```python
from build123d import *

# Parameters (mm, degrees)
SALIENTE_EXTRUIR1_DEPTH = 10
REDONDEO1_R             = 2
CROQUIS4_R              = 1.75
SALIENTE_EXTRUIR2_DEPTH = 2
REDONDEO3_R             = 1
REDONDEO4_R             = 0.9


with BuildPart() as part:
    # Croquis2 → Saliente-Extruir1 (new body)
    with BuildSketch(Plane.XY):
        with BuildLine():
            Line((-10.4, 0), (10.4, 0))
            Line((10.4, 0), (10.4, 38))
            Line((10.4, 38), (6.4, 38))
            Line((6.4, 38), (6.4, 36))
            ThreePointArc((6.4, 36), (7.814213562, 35.414213562), (8.4, 34))
            Line((8.4, 34), (8.4, 1.5))
            Line((8.4, 1.5), (-8.4, 1.5))
            Line((-8.4, 1.5), (-8.4, 34))
            ThreePointArc((-8.4, 34), (-7.814213562, 35.414213562), (-6.4, 36))
            Line((-6.4, 36), (-6.4, 38))
            Line((-6.4, 38), (-10.4, 38))
            Line((-10.4, 38), (-10.4, 0))
        make_face()
    extrude(amount=SALIENTE_EXTRUIR1_DEPTH)

    # Redondeo1
    redondeo1_edges = [part.edges().sort_by_distance(p)[0] for p in [
        (-8.4, 1.5, 5),
        (8.4, 1.5, 5),
    ]]
    fillet(redondeo1_edges, radius=REDONDEO1_R)

    # Croquis4 → Saliente-Extruir2 (add)
    # profile 1 of 2: a face of its own
    with BuildSketch(Plane.XZ):
        with BuildLine():
            Line((-10.4, 10), (-15.4, 10))
            ThreePointArc((-15.4, 10), (-20.4, 5), (-15.4, 0))
            Line((-15.4, 0), (-10.4, 0))
            Line((-10.4, 0), (-10.4, 10))
        make_face()
        with Locations((-15.4, 5)):
            Circle(CROQUIS4_R, mode=Mode.SUBTRACT)
    # profile 2 of 2: a face of its own
    with BuildSketch(Plane.XZ):
        with BuildLine():
            Line((10.4, 0), (15.4, 0))
            ThreePointArc((15.4, 0), (20.4, 5), (15.4, 10))
            Line((15.4, 10), (10.4, 10))
            Line((10.4, 10), (10.4, 0))
        make_face()
        with Locations(Location((15.4, 5, 0), (0, 0, 180))):
            Circle(CROQUIS4_R, mode=Mode.SUBTRACT)
    extrude(amount=-SALIENTE_EXTRUIR2_DEPTH)

    # Redondeo3
    redondeo3_edges = [part.edges().sort_by_distance(p)[0] for p in [
        (-10.4, 2, 5),
        (10.4, 2, 5),
    ]]
    fillet(redondeo3_edges, radius=REDONDEO3_R)

    # Redondeo4
    redondeo4_edges = [part.edges().sort_by_distance(p)[0] for p in [
        (-10.4, 20.5, 0),
        (-7.814213562, 35.414213562, 0),
        (8.4, 18.75, 0),
        (7.814213562, 35.414213562, 0),
        (7.814213562, 35.414213562, 10),
        (8.4, 18.75, 10),
        (-7.814213562, 35.414213562, 10),
        (0, 1.5, 0),
        (0, 1.5, 10),
        (-8.4, 18.75, 0),
        (-8.4, 18.75, 10),
        (-8.4, 38, 10),
        (7.814213562, 2.085786438, 0),
        (7.814213562, 2.085786438, 10),
        (-7.814213562, 2.085786438, 0),
        (-7.814213562, 2.085786438, 10),
        (-10.4, 20.5, 10),
        (-13.4, 2, 0),
        (-20.4, 2, 5),
        (13.4, 2, 10),
        (20.4, 2, 5),
        (10.4, 20.5, 10),
        (10.4, 20.5, 0),
        (13.4, 2, 0),
        (-13.4, 2, 10),
        (10.692893219, 2.292893219, 0),
        (10.692893219, 2.292893219, 10),
        (-10.692893219, 2.292893219, 10),
        (-10.692893219, 2.292893219, 0),
        (8.4, 38, 10),
    ]]
    fillet(redondeo4_edges, radius=REDONDEO4_R)


solid = part.part
```
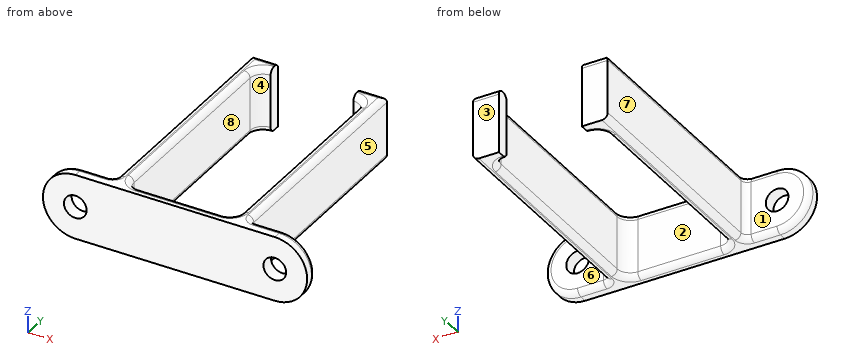
Here's how the part is built. I have some questions about the finished solid (model axes, mm). Face numbers are marked on the shaded views. A direction names the side the tool comes from. Give positions to 0.01 mm unless a question says otherwise; leave off trailing zeros. Loops run counter-clockwise (first coordinate to the right, second up) from the corner with the lowest first, then second, coordinate; pieces in that order, holes last. Notation, with made-up numbers: M -2.5,-10 L 48.5,-10 A23 ccw 48.5,26 Z; hole C -8.5,-1.75 d3. An arc over 180 degrees is marked long. Return JSON: item names as keys, results as strings.
Item 1: Imagine slicing it at A-A on y = 6.5. List the corners of the cut face in (x, z) for me.
A:
{"outline": "M -10.4,0.9 A0.9 ccw -9.5,0 L -9.3,0 A0.9 ccw -8.4,0.9 L -8.4,9.1 A0.9 ccw -9.3,10 L -9.5,10 A0.9 ccw -10.4,9.1 Z; M 8.4,0.9 A0.9 ccw 9.3,0 L 9.5,0 A0.9 ccw 10.4,0.9 L 10.4,9.1 A0.9 ccw 9.5,10 L 9.3,10 A0.9 ccw 8.4,9.1 Z"}
Item 2: Thinking about a two-plate mould opening in Y: for the marked faces 6, 7 and 8, which applies, released by +Y, released by -Y, zero draft, split by the parting line, or undercut?
A:
{"face 6": "released by +Y", "face 7": "zero draft", "face 8": "undercut"}
Item 3: On a 3-axis mill with a long thin cutter (end or side, diameter ignored), from which of +Z, -Z, +X, -X, +Y, -Y can I reach the whole of each face in a straight line? I mean the marked faces 1, 2, 3, 4 and 5. Say none if no direction works.
A:
{"face 1": "+Z, -Z, -X, +Y", "face 2": "+Z, -Z, +Y", "face 3": "+Z, -Z, +X, -X, +Y", "face 4": "+Z, -Z", "face 5": "+Z, -Z, +X, +Y"}
Item 4: Imagine slicing it at D-D on x = 4.5. List the corners of the cut face in (y, z) for me.
A:
{"outline": "M 0,0 L 0.6,0 A0.9 ccw 1.5,0.9 L 1.5,9.1 A0.9 ccw 0.6,10 L 0,10 Z"}
Item 5: Imagine slicing it at C-C on x = 12. List the corners of the cut face in (y, z) for me.
A:
{"outline": "M 0,0 L 1.1,0 A0.9 ccw 2,0.9 L 2,9.1 A0.9 ccw 1.1,10 L 0,10 Z"}
Item 6: Imagine slicing it at B-B on z = 5. State how many separate pieces and enclosed holes the cut face has, then the cut area to 3 significant figures.
A:
{"separate pieces": "3", "enclosed holes": "0", "area": "215 mm^2"}
Item 7: Please list where these lines run through material, in increasing order: line 1 (X direction, y = 17, z = 3.5); line 2 (Z direction, x = 15.4, y = 1); line 3 (Y direction, x = 6.5, z = 7.25).
A:
{"line 1": "x = -10.4 to -8.4, 8.4 to 10.4", "line 2": "z = 0 to 3.25, 6.75 to 10", "line 3": "y = 0 to 1.5, 36 to 38"}
Item 8: I'm going to push flat-ended pins straight in: pin 1 Ø4 at (y, z) = (19, 4.5) entering from +X; pin 2 Ø2.5 at (y, z) = (11.5, 3.5) entering from -X; pin 3 Ø2 at (x, z) = (15.4, 5) entering from -Y; pin 4 Ø1.5 at (x, z) = (-1, 6) entering from +Y. Where does each tip first touch, or does it pass through?
A:
{"pin 1": "stops at x = 10.4", "pin 2": "stops at x = -10.4", "pin 3": "passes through", "pin 4": "stops at y = 1.5"}
